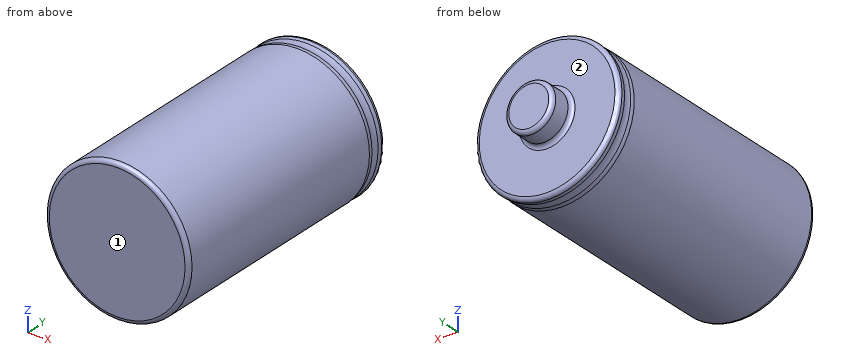
```python
from build123d import *

# Parameters (mm, degrees)
FILLET1_R = 0.5


with BuildPart() as part:
    # Sketch1 → Revolve1 (revolve)
    with BuildSketch(Plane.XY, mode=Mode.PRIVATE) as revolve1_sk:
        Polygon((0, -17.5), (0, 17.5), (3, 17.5), (3, 14.5), (9, 14.5), (9, -17.5), align=None)
    revolve(revolve1_sk.sketch.rotate(Axis((0, -17.5, 0), (0, 1, 0)), 90), axis=Axis((0, -17.5, 0), (0, 1, 0)))

    # Fillet1
    fillet1_edges = [part.edges().sort_by_distance(p)[0] for p in [
        (0, -17.5, 9),
        (0, 14.5, 9),
        (0, 14.5, 3),
        (0, 17.5, 3),
    ]]
    fillet(fillet1_edges, radius=FILLET1_R)

    # Sketch2 → Cut-Revolve1 (revolve, cut)
    with BuildSketch(Plane.XY, mode=Mode.PRIVATE) as cut_revolve1_sk:
        with BuildLine():
            Line((9, 12), (9, 14))
            ThreePointArc((9, 14), (8.984059393, 13.747991415), (8.936491673, 13.5))
            ThreePointArc((8.936491673, 13.5), (8.872983346, 13), (8.936491673, 12.5))
            ThreePointArc((8.936491673, 12.5), (8.984059393, 12.252008585), (9, 12))
        make_face()
    revolve(cut_revolve1_sk.sketch.rotate(Axis((0, 17.5, 0), (0, -1, 0)), 90), axis=Axis((0, 17.5, 0), (0, -1, 0)), mode=Mode.SUBTRACT)


solid = part.part
```
CAD build for the part. Positions are in the model's coordinates, mm. Face numbers are marked on the shaded views. A direction names the side the tool comes from. Coordinates: 2 decimals unless noted, no trailing zeros. Order: outer loops, then holes, each group sorted by start corner. A loop starts at its lowest first (then second) coordinate and runs counter-clockwise, first axis right, second up. Notation, with made-up numbers: (42, 66) -> (62, 66) arc R31 ccw to (62, 100) -> close; hole circle Ø9 at (24.5, 35.25). An arc over 180 degrees is marked (long way). Use one line per item in the form item = value. Start each with the question number.
1) Band-saw the part on B-B on x = 0. Give the cut face in (y, z), then the cut area to 3 significant figures.
2) Drill centre lines: L1, parallel to Y at x = -4.25, z = -2.25; L2, parallel to Z at x = 1, y = -0.5. Where is each one in solid material? Low to high. Write a range as [from, to].
3) Band-saw the part on C-C on y = 1. Give the cut face in (x, z).
4) Band-saw the part on A-A on z = 0. Give the cut face in (x, y).
5) Tool access for the marked faces 1 and 2: list every direction of +Z, -Z, +X, -X, +Y, -Y with a clear straight run to the whole face (end or side of a thin tool).
6) Drop flat-ended pins along their axis: pin 1 (4 mm diameter, centred on y = -5.5, z = 6, fed in from +X); pin 2 (4 mm diameter, centred on y = 0, z = 2.5, fed in from +X); pin 3 (5 mm diameter, centred on x = -3.5, z = -4.5, fed in from +Y). Give the stop position or say it passes through.
Entries:
q1.outline = (-17.5, -8.5) arc R0.5 ccw to (-17, -9) -> (12, -9) arc R2 ccw to (12.5, -8.94) arc R2 cw to (13.5, -8.94) arc R2 ccw to (14, -9) arc R0.5 ccw to (14.5, -8.5) -> (14.5, -3.5) arc R0.5 cw to (15, -3) -> (17, -3) arc R0.5 ccw to (17.5, -2.5) -> (17.5, 2.5) arc R0.5 ccw to (17, 3) -> (15, 3) arc R0.5 cw to (14.5, 3.5) -> (14.5, 8.5) arc R0.5 ccw to (14, 9) arc R2 ccw to (13.5, 8.94) arc R2 cw to (12.5, 8.94) arc R2 ccw to (12, 9) -> (-17, 9) arc R0.5 ccw to (-17.5, 8.5) -> close
q1.area = 594 mm2
q2.L1 = [-17.5, 14.5]
q2.L2 = [-8.94, 8.94]
q3.outline = circle Ø18 at (0, 0)
q4.outline = (-9, -17) arc R0.5 ccw to (-8.5, -17.5) -> (8.5, -17.5) arc R0.5 ccw to (9, -17) -> (9, 12) arc R2 ccw to (8.94, 12.5) arc R2 cw to (8.94, 13.5) arc R2 ccw to (9, 14) arc R0.5 ccw to (8.5, 14.5) -> (3.5, 14.5) arc R0.5 cw to (3, 15) -> (3, 17) arc R0.5 ccw to (2.5, 17.5) -> (-2.5, 17.5) arc R0.5 ccw to (-3, 17) -> (-3, 15) arc R0.5 cw to (-3.5, 14.5) -> (-8.5, 14.5) arc R0.5 ccw to (-9, 14) arc R2 ccw to (-8.94, 13.5) arc R2 cw to (-8.94, 12.5) arc R2 ccw to (-9, 12) -> close
q5.face_1 = +Z, -Z, +X, -X, -Y
q5.face_2 = +Y
q6.pin_1 = 8.06
q6.pin_2 = 8.99
q6.pin_3 = 14.6
